Here's the drawing with two shaded views (mm, measured from the low corner). I have some questions. A direction names the side the tool comes from. Give positions to 0.01 mm unless a question says otherwise; leave off trailing zeros. Loops run counter-clockwise (first coordinate to the right, second up) from the corner with the lowest first, then second, coordinate; pieces in that order, holes last. Notation, with made-up numbers: (73, -16) - (108, -16) arc R25 ccw to (108, 0) - close; hole circle Ø10 at (-20, -26). An arc over 180 degrees is marked (long way). Answer as a JSON object with one key per item and string values. Group by question number.
Item 1: Suppose I cut it at B-B on y = 83. Write out the boundary of the cut face in (x, z).
Item 2: Thinking about a two-plate mould opening in Z: for the marked faces 1, 2, 3 and 4, which applies, pulls with the +Z half, pulls with the -Z half, needs draft (parallel to the pull), parting line crosses it, or undercut?
Item 3: Suppose I cut it at C-C on z = 86. Write out the boundary of the cut face in (x, y).
Item 4: Which directions (+Z, -Z, +X, -X, +Y, -Y) give clear straight access to the entire face, cutting with the end or side of a thin tool? Please do the marked faces 5 and 6.
Item 5: Will this pin go through, and if not, where does the flat tip stop? pin 1 (4 mm diameter, centred on x = 78, z = 75.5, fed in from -Y).
Item 6: Please list where these lines run through material, in increasing order: L1, parallel to X at y = 80.5, z = 130; L2, parallel to Z at x = 142.5, y = 86.5; L3, parallel to Z at x = 168, y = 49.
Item 7: Suppose I cut it at D-D on y = 26. Write out the boundary of the cut face in (x, z) (1 decimal), and give its area (3 significant figures).
Item 8: Suppose I cut it at A-A on x = 155.5. Write out the boundary of the cut face in (y, z) (1 decimal), and give its area (3 significant figures).
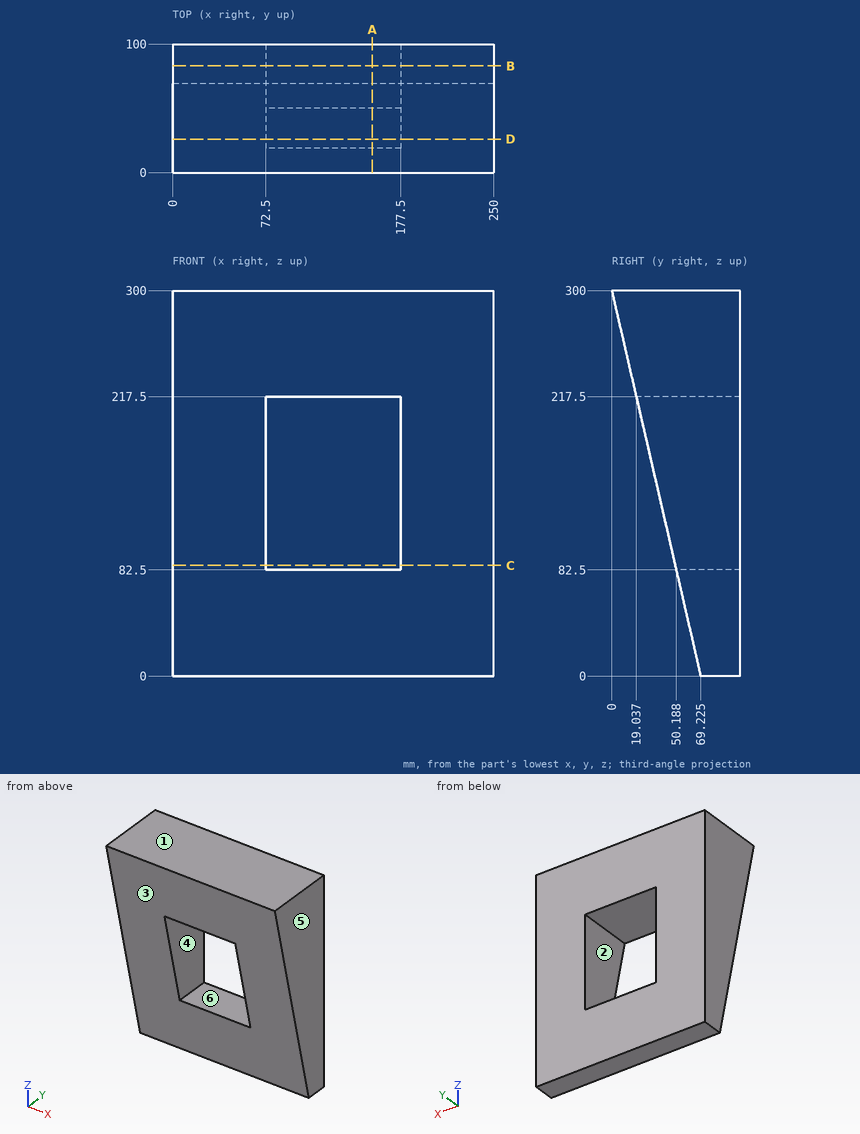
Worked out:
{
 "1": {"outline": "(0, 0) - (250, 0) - (250, 300) - (0, 300) - close; hole (72.5, 82.5) - (177.5, 82.5) - (177.5, 217.5) - (72.5, 217.5) - close"},
 "2": {"face 1": "pulls with the +Z half", "face 2": "undercut", "face 3": "pulls with the -Z half", "face 4": "undercut"},
 "3": {"outline": "(0, 49.38) - (72.5, 49.38) - (72.5, 100) - (0, 100) - close; (177.5, 49.38) - (250, 49.38) - (250, 100) - (177.5, 100) - close"},
 "4": {"face 5": "+Z, -Z, +X, +Y, -Y", "face 6": "+Y, -Y"},
 "5": {"pin 1": "stops at y = 51.34"},
 "6": {"L1": "x = 0 to 72.5, 177.5 to 250", "L2": "z = 0 to 82.5, 217.5 to 300", "L3": "z = 217.5 to 300"},
 "7": {"outline": "(0, 187.3) - (72.5, 187.3) - (72.5, 217.5) - (177.5, 217.5) - (177.5, 187.3) - (250, 187.3) - (250, 300) - (0, 300) - close", "area": "25,000 mm2"},
 "8": {"outline": "(0, 300) - (19, 217.5) - (100, 217.5) - (100, 300) - close; (50.2, 82.5) - (69.2, 0) - (100, 0) - (100, 82.5) - close", "area": "10,800 mm2"}
}
